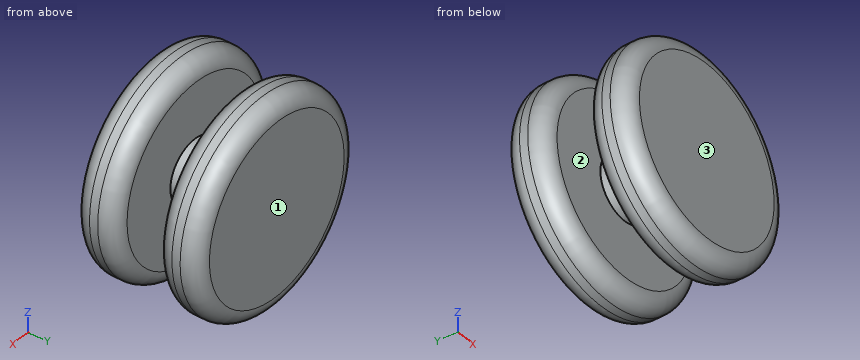
```python
from build123d import *

# Parameters (mm, degrees)
F0_R     = 31.75
F1_DEPTH = 12.7
F2_R     = 5.08
F3_R     = 9.525
F4_DEPTH = 6.35
F7_D     = 2.54
F7_DEPTH = 25.4
F7_TIP   = 0.7630929862


with BuildPart() as f1:
    # F0 (on Front) → F1 (new body)
    with BuildSketch(Plane.XZ):
        Circle(F0_R)
    extrude(amount=F1_DEPTH)

    # F2
    f2_edges = [f1.edges().sort_by_distance(p)[0] for p in [
        (-31.75, -12.7, 0),
        (-31.75, 0, 0),
    ]]
    fillet(f2_edges, radius=F2_R)

    # F3 (on face) → F4 (join)
    with BuildSketch(Plane(origin=(0, 0, 0), x_dir=(-1, 0, 0), z_dir=(0, 1, 0))):
        Circle(F3_R)
    extrude(amount=F4_DEPTH)

    # F5: F1 across face


with BuildPart() as f1_1:
    add(f1.part)
    add(f1.part.mirror(Plane(origin=(0, 6.35, 0), x_dir=(-1, 0, 0), z_dir=(0, 1, 0))))

    # F7 (one way)
    with BuildSketch(Plane.XY):
        with Locations((0, 6.0745161027)):
            Circle(F7_D / 2)
    extrude(amount=-F7_DEPTH, mode=Mode.SUBTRACT)
    with Locations(Plane.XY):
        with Locations((0, 6.0745161027)):
            with Locations((0, 0, -(F7_DEPTH + F7_TIP / 2))):  # 118° drill point
                Cone(0, F7_D / 2, F7_TIP, mode=Mode.SUBTRACT)


solid = f1_1.part
```
Verification items for the finished model (mm, model axes). Face numbers are marked on the shaded views. Round coordinates to 2 decimals unless told otherwise and drop trailing zeros. Order: outer loops, then holes, each group sorted by start corner. A loop starts at its lowest first (then second) coordinate and runs counter-clockwise, first axis right, second up. Notation, with made-up numbers: (83.5, 6.5) - (118.5, 6.5) arc R28 ccw to (118.5, 41.5) - close; hole circle Ø11 at (47.5, 20.5). An arc over 180 degrees is marked (long way). Use CSV: the item, a comma, the result in double quotes.
(1) Section check C-C on y = -3. Record the boundary of the cut face in (x, z).
Entries:
outline,"circle Ø62.61 at (0, 0)"
(2) Thickness scan on probe 1 along Y at (x, z) = (0, -5); probe 2 along Y at (x, z) = (9.5, 7.5); probe 3 along X at (y, z) = (9, -6). Record the ranges inside material, lowest first. Write a range as from..to.
Entries:
probe 1,"-12.7..4.8, 7.34..25.4"
probe 2,"-12.7..0, 12.7..25.4"
probe 3,"-7.4..7.4"
(3) Mould release check, pull along Y, two halves, no side actions. Record for the marked faces 1, 2 and 3: released by +Y, released by -Y, zero draft, split by the parting line, or undercut.
Entries:
face 1,"released by +Y"
face 2,"undercut"
face 3,"released by -Y"
(4) Section check B-B on y = 10. Record the boundary of the cut face in (x, z) (3 decimals).
Entries:
outline,"circle Ø19.05 at (0, 0)"
(5) Gauge pin test, flat ends, axial feed: pin 1 Ø5 at (x, y) = (-2, 19) entering from +Z; pin 2 Ø10 at (y, z) = (-4, 21) entering from -X; pin 3 Ø12 at (x, y) = (1.5, 11.5) entering from -Z. Record the tip position at first contact, or that the pin passes through.
Entries:
pin 1,"z = 31.75"
pin 2,"x = -27.38"
pin 3,"z = -31.73"
(6) Section check A-A on x = 0. Record the boundary of the cut face in (y, z) (3 decimals).
Entries:
outline,"(-12.7, -26.67) arc R5.08 ccw to (-7.62, -31.75) - (-5.08, -31.75) arc R5.08 ccw to (0, -26.67) - (0, -9.525) - (4.805, -9.525) - (4.805, 0) - (7.345, 0) - (7.345, -9.525) - (12.7, -9.525) - (12.7, -26.67) arc R5.08 ccw to (17.78, -31.75) - (20.32, -31.75) arc R5.08 ccw to (25.4, -26.67) - (25.4, 26.67) arc R5.08 ccw to (20.32, 31.75) - (17.78, 31.75) arc R5.08 ccw to (12.7, 26.67) - (12.7, 9.525) - (0, 9.525) - (0, 26.67) arc R5.08 ccw to (-5.08, 31.75) - (-7.62, 31.75) arc R5.08 ccw to (-12.7, 26.67) - close"
